```python
from build123d import *

# Parameters (mm, degrees)
F0_W     = 25.4
F0_H     = 50.8
F2_W     = 15.24
F2_H     = 40.64
F5_R     = 4.7625
F6_DEPTH = 50.801
F7_W     = 20.32
F7_H     = 45.72
F8_DEPTH = 1.5875


with BuildPart() as f3:
    # F0 (on Front) → F3 section 0
    with BuildSketch(Plane.XZ):
        Rectangle(F0_W, F0_H)
    # F2 (on offset) → F3 section 1
    with BuildSketch(Plane.XZ.offset(19.05)):
        Rectangle(F2_W, F2_H)
    loft()

    # F5 (on face) → F6 (cut, through all)
    with BuildSketch(Plane.XY.offset(25.4)):
        with Locations((0, -18.25625)):
            Circle(F5_R)
    extrude(amount=-F6_DEPTH, mode=Mode.SUBTRACT)

    # F7 (on face) → F8 (cut)
    with BuildSketch(Plane(origin=(0, 0, 0), x_dir=(-1, 0, 0), z_dir=(0, 1, 0))):
        Rectangle(F7_W, F7_H)
    extrude(amount=-F8_DEPTH, mode=Mode.SUBTRACT)


solid = f3.part
```
Could you check a few things on this model? Use its own coordinates, in mm. A direction names the side the tool comes from. Round coordinates to 2 decimals unless told otherwise and drop trailing zeros.
Q1. Thinking about a two-plate mould opening in X: for faces 3 (the flat face through (11, 0, -1)), 4 (the flat face through (-10.16, -1, 0)), 5 (the flat face through (0, -1, -22.86)), which applies, pulls with the +X half, pulls with the -X half, needs draft (parallel to the pull), parting line crosses it, or undercut?
Q2. Please list where these lines run through material, in increasing order: L1, parallel to Y at x = 5, z = -8.5; L2, parallel to Y at x = 0, z = -3.5; L3, parallel to X at y = -17.5, z = 5.5.
Q3. For P1, Ø0.8, axis at y = -1, z = -7.5, coming from the -X side; P2, Ø2, axis at y = -16.5, z = -9, coming from the -X side; P3, Ø10, axis at x = 4, z = 5, coming from the +Y side, each with a flat end and sliding along its axis, tell me the tip position at first contact or that it passes through.
Q4. On a 3-axis mill with a long thin cutter (end or side, diameter ignored), from which of +Z, -Z, +X, -X, +Y, -Y can I reach the whole of each face in a straight line? I mean faces 1 (the flat face through (0, -1, 22.86)), 2 (the flat face through (6, -19.05, 0)). Say none if no direction works.
Answer below:
1. face 3: needs draft
1. face 4: undercut
1. face 5: undercut
2. L1: y = -19.05 to -1.59
2. L2: y = -13.49 to -1.59
2. L3: x = -8.03 to -4.7, 4.7 to 8.03
3. P1: stops at x = -12.54
3. P2: stops at x = -8.57
3. P3: stops at y = -1.59
4. face 1: +Y
4. face 2: +Z, -Z, +X, -X, -Y
